```python
from build123d import *

# Parameters (mm, degrees)
SKETCH_1_R      = 1.6
EXTRUDE_1_DEPTH = 3
FILLET_1_R      = 3
FILLET_2_R      = 15


with BuildPart() as part:
    # 草图1 → 凸台-拉伸1 (new body)
    with BuildSketch(Plane.XY):
        Polygon((0, 0), (40, 0), (40, -40), (20, -40), (20, -20), (0, -20), align=None)
        with Locations((5, -5)):
            Circle(SKETCH_1_R, mode=Mode.SUBTRACT)
        with Locations(Location((15, -5, 0), (0, 0, 180))):
            Circle(SKETCH_1_R, mode=Mode.SUBTRACT)
        with Locations((15, -15)):
            Circle(SKETCH_1_R, mode=Mode.SUBTRACT)
        with Locations(Location((5, -15, 0), (0, 0, 180))):
            Circle(SKETCH_1_R, mode=Mode.SUBTRACT)
        with Locations((25, -35)):
            Circle(SKETCH_1_R, mode=Mode.SUBTRACT)
        with Locations(Location((35, -35, 0), (0, 0, 180))):
            Circle(SKETCH_1_R, mode=Mode.SUBTRACT)
        with Locations((35, -25)):
            Circle(SKETCH_1_R, mode=Mode.SUBTRACT)
        with Locations(Location((25, -25, 0), (0, 0, 180))):
            Circle(SKETCH_1_R, mode=Mode.SUBTRACT)
        Polygon((23, -5), (23, -15), (33, -15), align=None, mode=Mode.SUBTRACT)
        Polygon((27, -5), (37, -5), (37, -15), align=None, mode=Mode.SUBTRACT)
    extrude(amount=EXTRUDE_1_DEPTH)

    # 圆角1
    fillet_1_edges = [part.edges().sort_by_distance(p)[0] for p in [
        (0, 0, 1.5),
        (40, 0, 1.5),
        (40, -40, 1.5),
        (20, -40, 1.5),
        (0, -20, 1.5),
    ]]
    fillet(fillet_1_edges, radius=FILLET_1_R)

    # 圆角2
    fillet_2_edges = [part.edges().sort_by_distance(p)[0] for p in [
        (20, -20, 1.5),
    ]]
    fillet(fillet_2_edges, radius=FILLET_2_R)


solid = part.part
```
Input: part model. Units: mm. Frame: model coordinates. A direction names the side the tool comes from. Give positions to 0.01 mm unless a question says otherwise; leave off trailing zeros. Loops run counter-clockwise (first coordinate to the right, second up) from the corner with the lowest first, then second, coordinate; pieces in that order, holes last.
1) Contact query for flat-ended pins moving along their axis: pin 1 (1.5 mm diameter, centred on x = 16, z = 1, fed in from -Y); pin 2 (0.6 mm diameter, centred on x = 4, z = 1.5, fed in from -Y); pin 3 (1 mm diameter, centred on y = -36, z = 1, fed in from -X). Output: stop coordinate, or through.
A:
pin 1: stops at y = -25.68
pin 2: stops at y = -20
pin 3: stops at x = 20
2) Line query: L1, parallel to X at y = -10.5, z = 1.05; L2, parallel to Y at x = 15, z = 2; L3, parallel to Y at x = 25, z = 0.9. Output: solid intervals per line, ascending.
A:
L1: x = 0 to 23, 28.5 to 32.5, 37 to 40
L2: y = -23.82 to -16.6, -13.4 to -6.6, -3.4 to 0
L3: y = -40 to -36.6, -33.4 to -26.6, -23.4 to -15, -7 to 0
3) Mould query, pull axis X, two halves, no side actions, for faces 4 (the flat face through (20, -36, 1)), 5 (the cylindrical face through (39.14, -39.1, 1.52)), 6 (the cylindrical face through (26.27, -24.03, 1.48)). Classes: released by +X, released by -X, zero draft, split by the parting line, or undercut.
A:
face 4: released by -X
face 5: released by +X
face 6: undercut
4) Section query B-B on y = -10. Return the cut outline in (x, z), and give its area (3 significant figures).
A:
outline: (0, 0) - (23, 0) - (23, 3) - (0, 3) - close; (28, 0) - (32, 0) - (32, 3) - (28, 3) - close; (37, 0) - (40, 0) - (40, 3) - (37, 3) - close
area: 90.0 mm2
5) Reachability of faces 1 (the flat face through (37, -10, 1)), 2 (the flat face through (40, -20, 1)), 3 (the flat face through (4, -20, 1)) from +Z, -Z, +X, -X, +Y, -Y: full face, straight path, thin tool, end or side. Return the list, or none.
A:
face 1: +Z, -Z
face 2: +Z, -Z, +X, +Y, -Y
face 3: +Z, -Z, -X, -Y
6) Section query A-A on x = 25. Return the cut outline in (y, z).
A:
outline: (-40, 0) - (-36.6, 0) - (-36.6, 3) - (-40, 3) - close; (-33.4, 0) - (-26.6, 0) - (-26.6, 3) - (-33.4, 3) - close; (-23.4, 0) - (-15, 0) - (-15, 3) - (-23.4, 3) - close; (-7, 0) - (0, 0) - (0, 3) - (-7, 3) - close
7) Section query C-C on z = 1.7. Count the separate pieces of the cut face and the enclosed holes in it, and give its area (3 significant figures).
A:
separate pieces: 1
enclosed holes: 10
area: 1,070 mm2
8) Section query D-D on x = 15. Return the cut outline in (y, z), and give its area (3 significant figures).
A:
outline: (-23.82, 0) - (-16.6, 0) - (-16.6, 3) - (-23.82, 3) - close; (-13.4, 0) - (-6.6, 0) - (-6.6, 3) - (-13.4, 3) - close; (-3.4, 0) - (0, 0) - (0, 3) - (-3.4, 3) - close
area: 52.3 mm2
